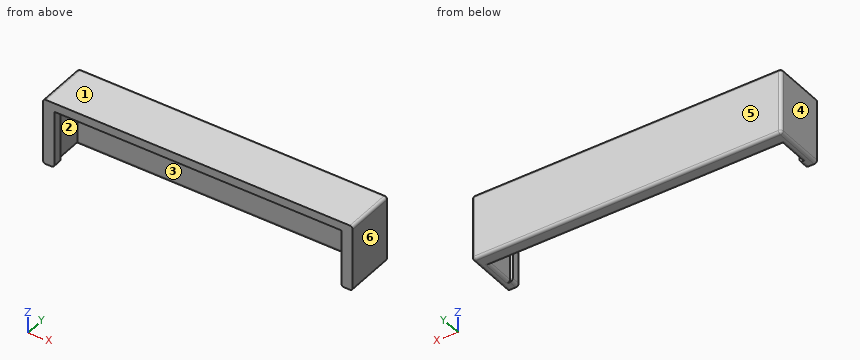
from build123d import *

# Parameters (mm, degrees)
F0_W     = 1
F0_H     = 20
F0_W_2   = 100
F1_DEPTH = 18
F2_DEPTH = 13
F3_DEPTH = 3
F4_R     = 0.9999


# Not quite as in the source:
# - a fillet or chamfer is up to 0.001 mm smaller than in the source, because OpenCascade refuses the exact size


with BuildPart() as f1:
    # F0 (on Front) → F1 (new body)
    with BuildSketch(Plane.XZ):
        Polygon((51, 20), (51, 0), (54, 0), (54, 23), (-54, 23), (-54, 0), (-51, 0), (-51, 20), (-50, 20), (50, 20), align=None)
        with Locations((-50.5, 10)):
            Rectangle(F0_W, F0_H)
        with Locations((0, 10)):
            Rectangle(F0_W_2, F0_H)
        with Locations((50.5, 10)):
            Rectangle(F0_W, F0_H)
    extrude(amount=-F1_DEPTH)

    # F0 (on Front) → F2 (cut)
    with BuildSketch(Plane.XZ):
        with Locations((-50.5, 10)):
            Rectangle(F0_W, F0_H)
        with Locations((0, 10)):
            Rectangle(F0_W_2, F0_H)
        with Locations((50.5, 10)):
            Rectangle(F0_W, F0_H)
    extrude(amount=-F2_DEPTH, mode=Mode.SUBTRACT)

    # F0 (on Front) → F3 (join)
    with BuildSketch(Plane.XZ):
        with Locations((-50.5, 10)):
            Rectangle(F0_W, F0_H)
        with Locations((50.5, 10)):
            Rectangle(F0_W, F0_H)
    extrude(amount=-F3_DEPTH)

    # F4 (radius 1 in the source; OpenCascade refuses exactly that, so slightly less here)
    f4_edges = [f1.edges().sort_by_distance(p)[0] for p in [
        (-54, 18, 11.5),
        (54, 18, 11.5),
        (0, 18, 0),
        (54, 9, 0),
        (-54, 9, 0),
        (-54, 9, 23),
        (0, 18, 23),
        (54, 9, 23),
        (0, 13, 0),
        (51, 8, 0),
        (-51, 8, 0),
        (-50, 1.5, 0),
        (50, 1.5, 0),
    ]]
    fillet(f4_edges, radius=F4_R)


solid = f1.part
Check sheet for the modelled part. Datum: model origin and axes. Units: mm. Face numbers are marked on the shaded views. A direction names the side the tool comes from. Round coordinates to 2 decimals unless told otherwise and drop trailing zeros. Order: outer loops, then holes, each group sorted by start corner. A loop starts at its lowest first (then second) coordinate and runs counter-clockwise, first axis right, second up. Notation, with made-up numbers: M 56,19.25 L 110,19.25 A23 ccw 110,27.25 Z; hole C -13,32 d2. An arc over 180 degrees is marked long. One line per item, written item: value. Start each with the question number.
1. Section check B-B on y = 1.75. Enter the section's corners in (x, z), and give its area (3 significant figures).
2. Section check A-A on x = -24. Enter the section's corners in (y, z), and give its area (3 significant figures).
3. Section check C-C on z = 11. Enter the section's corners in (x, y), and give its area (3 significant figures).
4. Access from +Z, -Z, +X, -X, +Y, -Y to the whole of each face (thin tool, end or side, straight path). Record for the marked faces 1 and 2.
5. Gauge pin test, flat ends, axial feed: P1, Ø1.5, axis at x = -24, y = 6, coming from the -Z side; P2, Ø9.5, axis at x = -13, z = 12, coming from the -Y side. Record the tip position at first contact, or that the pin passes through.
6. Release check for a two-part mould opening along X. For the marked faces 3, 4, 5 and 6 record: released by +X, released by -X, zero draft, split by the parting line, or undercut.
7. Scan lines: line 1 along X through (y, z) = (8.5, 9); line 2 along Y through (x, z) = (28, 10.5); line 3 along Z through (x, y) = (9.5, 5). Record each from-to range of solid material in increasing order.
Results found:
1. outline: M -54,1 A1 ccw -53,0 L -51,0 A1 ccw -50,1 L -50,20 L 50,20 L 50,1 A1 ccw 51,0 L 53,0 A1 ccw 54,1 L 54,22 A1 ccw 53,23 L -53,23 A1 ccw -54,22 Z
1. area: 483 mm^2
2. outline: M 0,20 L 13,20 L 13,1 A1 ccw 14,0 L 17,0 A1 ccw 18,1 L 18,22 A1 ccw 17,23 L 0,23 Z
2. area: 153 mm^2
3. outline: M -54,0 L -50,0 L -50,3 L -51,3 L -51,13 L 51,13 L 51,3 L 50,3 L 50,0 L 54,0 L 54,17 A1 ccw 53,18 L -53,18 A1 ccw -54,17 Z
3. area: 624 mm^2
4. face 1: +Z, +X, -X, +Y, -Y
4. face 2: -Z
5. P1: z = 20
5. P2: y = 13
6. face 3: undercut
6. face 4: released by -X
6. face 5: zero draft
6. face 6: released by +X
7. line 1: -54 to -51, 51 to 54
7. line 2: 13 to 18
7. line 3: 20 to 23
